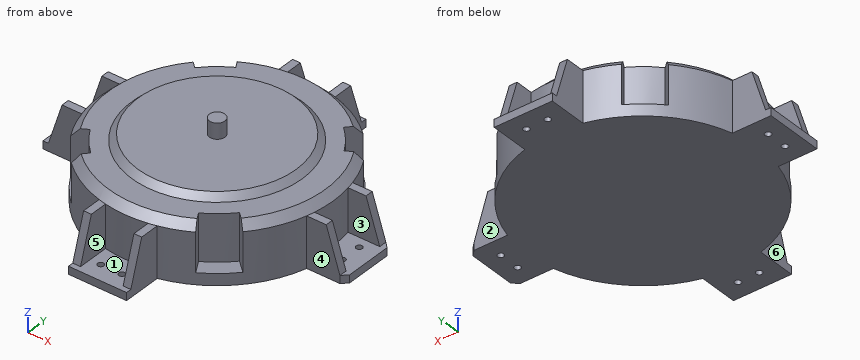
from build123d import *

# Parameters (mm, degrees)
IZIM1_R                           = 150
Y_KSEKLIK_EKSTR_ZYON1_DEPTH       = 75
PAH1_SIZE                         = 10
Y_KSEKLIK_EKSTR_ZYON2_START       = -75
Y_KSEKLIK_EKSTR_ZYON2_DEPTH       = 10
PAH2_SIZE                         = 7
Y_KSEKLIK_EKSTR_ZYON3_DEPTH       = 10
IZIM8_R                           = 4
KES_EKSTR_ZYON1_DEPTH             = 255.641782801
DAIRESEL_KAPLAMA1_COUNT           = 4
DAIRESEL_KAPLAMA1_COPY_1_DEPTH    = 10
DAIRESEL_KAPLAMA1_COPY_2_DEPTH    = 10
DAIRESEL_KAPLAMA1_COPY_3_DEPTH    = 10
DAIRESEL_KAPLAMA1_COPY_4_SKETCH_R = 4
DAIRESEL_KAPLAMA1_COPY_4_DEPTH    = 255.641782801
DAIRESEL_KAPLAMA1_COPY_5_SKETCH_R = 4
DAIRESEL_KAPLAMA1_COPY_5_DEPTH    = 255.641782801
DAIRESEL_KAPLAMA1_COPY_6_SKETCH_R = 4
DAIRESEL_KAPLAMA1_COPY_6_DEPTH    = 255.641782801
KES_EKSTR_ZYON2_START             = -60
KES_EKSTR_ZYON2_DEPTH             = 60
DAIRESEL_KAPLAMA2_COUNT           = 4
IZIM10_R                          = 110
Y_KSEKLIK_EKSTR_ZYON4_DEPTH       = 8
Y_KSEKLIK_EKSTR_ZYON4_TAPER       = 45
IZIM11_R                          = 10
Y_KSEKLIK_EKSTR_ZYON5_DEPTH       = 20


with BuildPart() as part:
    # Çizim1 → Yükseklik-Ekstrüzyon1 (new body)
    with BuildSketch(Plane.XY):
        Circle(IZIM1_R)
    extrude(amount=Y_KSEKLIK_EKSTR_ZYON1_DEPTH)

    # Pah1
    pah1_edges = [part.edges().sort_by_distance(p)[0] for p in [
        (-150, 0, 75),
    ]]
    chamfer(pah1_edges, length=PAH1_SIZE)

    # Çizim4 → Yükseklik-Ekstrüzyon2 (add)
    with BuildSketch(Plane.XY.offset(75).offset(Y_KSEKLIK_EKSTR_ZYON2_START)):
        with BuildLine():
            Line((195.236875483, -37.5), (195.236875483, 37.5))
            Line((195.236875483, 37.5), (145.236875483, 37.5))
            ThreePointArc((145.236875483, 37.5), (150, 0), (145.236875483, -37.5))
            Line((145.236875483, -37.5), (195.236875483, -37.5))
        make_face()
    y_kseklik_ekstr_zyon2 = extrude(amount=Y_KSEKLIK_EKSTR_ZYON2_DEPTH)

    # Pah2
    pah2_edges = [part.edges().sort_by_distance(p)[0] for p in [
        (195.236875483, -37.5, 5),
        (195.236875483, 37.5, 5),
    ]]
    chamfer(pah2_edges, length=PAH2_SIZE)

    # Çizim7 → Yükseklik-Ekstrüzyon3 (add)
    with BuildSketch(Plane(origin=(0, 37.5, 0), x_dir=(1, 0, 0), z_dir=(0, 1, 0))):
        Polygon((145.236875483, 0), (145.236875483, -65.015207496), (170.556875483, -65.015207496), (188.236875483, -10), (188.236875483, 0), align=None)
    y_kseklik_ekstr_zyon3 = extrude(amount=-Y_KSEKLIK_EKSTR_ZYON3_DEPTH)

    # Çizim8 → Kes-Ekstrüzyon1 (cut, through all)
    with BuildSketch(Plane.XY.offset(10)):
        with Locations((172.618437741, 13.75)):
            Circle(IZIM8_R)
    kes_ekstr_zyon1 = extrude(amount=-KES_EKSTR_ZYON1_DEPTH, mode=Mode.SUBTRACT)

    # Aynalama1: Yükseklik-Ekstrüzyon3, Kes-Ekstrüzyon1 across plane
    add(y_kseklik_ekstr_zyon3.mirror(Plane.ZX))
    add(kes_ekstr_zyon1.mirror(Plane.ZX), mode=Mode.SUBTRACT)

    # Dairesel Kaplama1: Yükseklik-Ekstrüzyon2, Yükseklik-Ekstrüzyon3, Kes-Ekstrüzyon1 ×4 about axis
    dairesel_kaplama1_axis = Axis((0, 0, 0), (0, 0, 1))
    add([y_kseklik_ekstr_zyon2.rotate(dairesel_kaplama1_axis, i * 360 / DAIRESEL_KAPLAMA1_COUNT) for i in range(1, DAIRESEL_KAPLAMA1_COUNT)])
    add([y_kseklik_ekstr_zyon3.rotate(dairesel_kaplama1_axis, i * 360 / DAIRESEL_KAPLAMA1_COUNT) for i in range(1, DAIRESEL_KAPLAMA1_COUNT)])
    add([kes_ekstr_zyon1.rotate(dairesel_kaplama1_axis, i * 360 / DAIRESEL_KAPLAMA1_COUNT) for i in range(1, DAIRESEL_KAPLAMA1_COUNT)], mode=Mode.SUBTRACT)

    # Dairesel Kaplama1 copy 1 sketch → Dairesel Kaplama1 copy 1 (add)
    with BuildSketch(Plane.YZ.offset(37.5)):
        Polygon((145.236875483, 0), (145.236875483, 65.015207496), (170.556875483, 65.015207496), (188.236875483, 10), (188.236875483, 0), align=None)
    extrude(amount=-DAIRESEL_KAPLAMA1_COPY_1_DEPTH)

    # Dairesel Kaplama1 copy 2 sketch → Dairesel Kaplama1 copy 2 (add)
    with BuildSketch(Plane(origin=(0, 37.5, 0), x_dir=(-1, 0, 0), z_dir=(0, 1, 0))):
        Polygon((145.236875483, 0), (145.236875483, 65.015207496), (170.556875483, 65.015207496), (188.236875483, 10), (188.236875483, 0), align=None)
    extrude(amount=-DAIRESEL_KAPLAMA1_COPY_2_DEPTH)

    # Dairesel Kaplama1 copy 3 sketch → Dairesel Kaplama1 copy 3 (add)
    with BuildSketch(Plane(origin=(-37.5, 0, 0), x_dir=(0, -1, 0), z_dir=(-1, 0, 0))):
        Polygon((145.236875483, 0), (145.236875483, 65.015207496), (170.556875483, 65.015207496), (188.236875483, 10), (188.236875483, 0), align=None)
    extrude(amount=-DAIRESEL_KAPLAMA1_COPY_3_DEPTH)

    # Dairesel Kaplama1 copy 4 sketch → Dairesel Kaplama1 copy 4 (cut, through all)
    with BuildSketch(Plane(origin=(0, 0, 10), x_dir=(0, 1, 0), z_dir=(0, 0, 1))):
        with Locations((172.618437741, -13.75)):
            Circle(DAIRESEL_KAPLAMA1_COPY_4_SKETCH_R)
    extrude(amount=-DAIRESEL_KAPLAMA1_COPY_4_DEPTH, mode=Mode.SUBTRACT)

    # Dairesel Kaplama1 copy 5 sketch → Dairesel Kaplama1 copy 5 (cut, through all)
    with BuildSketch(Plane(origin=(0, 0, 10), x_dir=(-1, 0, 0), z_dir=(0, 0, 1))):
        with Locations((172.618437741, -13.75)):
            Circle(DAIRESEL_KAPLAMA1_COPY_5_SKETCH_R)
    extrude(amount=-DAIRESEL_KAPLAMA1_COPY_5_DEPTH, mode=Mode.SUBTRACT)

    # Dairesel Kaplama1 copy 6 sketch → Dairesel Kaplama1 copy 6 (cut, through all)
    with BuildSketch(Plane(origin=(0, 0, 10), x_dir=(0, -1, 0), z_dir=(0, 0, 1))):
        with Locations((172.618437741, -13.75)):
            Circle(DAIRESEL_KAPLAMA1_COPY_6_SKETCH_R)
    extrude(amount=-DAIRESEL_KAPLAMA1_COPY_6_DEPTH, mode=Mode.SUBTRACT)

    # Çizim9 → Kes-Ekstrüzyon2 (cut)
    with BuildSketch(Plane.XY.offset(75).offset(KES_EKSTR_ZYON2_START)):
        with BuildLine():
            Line((-112.583302492, -65), (-129.903810568, -75))
            ThreePointArc((-129.903810568, -75), (-116.277268219, -94.760734988), (-99.673152863, -112.094882124))
            Line((-99.673152863, -112.094882124), (-86.383399148, -97.148897841))
            ThreePointArc((-86.383399148, -97.148897841), (-100.773632456, -82.125970323), (-112.583302492, -65))
        make_face()
    kes_ekstr_zyon2 = extrude(amount=KES_EKSTR_ZYON2_DEPTH, mode=Mode.SUBTRACT)

    # Dairesel Kaplama2: Kes-Ekstrüzyon2 ×4 about axis
    dairesel_kaplama2_axis = Axis((0, 0, 75), (0, 0, 1))
    for i in range(1, DAIRESEL_KAPLAMA2_COUNT):
        add(kes_ekstr_zyon2.rotate(dairesel_kaplama2_axis, i * 360 / DAIRESEL_KAPLAMA2_COUNT), mode=Mode.SUBTRACT)

    # Çizim10 → Yükseklik-Ekstrüzyon4 (add)
    with BuildSketch(Plane.XY.offset(75)):
        Circle(IZIM10_R)
    extrude(amount=Y_KSEKLIK_EKSTR_ZYON4_DEPTH, taper=Y_KSEKLIK_EKSTR_ZYON4_TAPER)

    # Çizim11 → Yükseklik-Ekstrüzyon5 (add)
    with BuildSketch(Plane.XY.offset(83)):
        Circle(IZIM11_R)
    extrude(amount=Y_KSEKLIK_EKSTR_ZYON5_DEPTH)


solid = part.part
Verification items for the finished model (mm, model axes). Face numbers are marked on the shaded views. A direction names the side the tool comes from. Round coordinates to 2 decimals unless told otherwise and drop trailing zeros. Loops run counter-clockwise (first coordinate to the right, second up) from the corner with the lowest first, then second, coordinate; pieces in that order, holes last. Notation, with made-up numbers: (38, 16) - (66, 16) arc R19 ccw to (66, 30) - close; hole circle Ø3 at (-28.75, -10). An arc over 180 degrees is marked (long way). Write item = value, one per line.
Q1. Sectioned sample at A-A on y = 0. Record the boundary of the cut face in (x, z), plus the area to 3 significant figures.
Here are the results:
outline = (-195.24, 0) - (195.24, 0) - (195.24, 10) - (150, 10) - (150, 65) - (140, 75) - (110, 75) - (102, 83) - (10, 83) - (10, 103) - (-10, 103) - (-10, 83) - (-102, 83) - (-110, 75) - (-140, 75) - (-150, 65) - (-150, 10) - (-195.24, 10) - close
area = 25,400 mm^2
Q2. Material ranges on L1, parallel to Y at x = 13.75, z = 3.5; L2, parallel to X at y = 166, z = 26.5; L3, parallel to Z at x = 91, y = -104.5, recorded low to high.
Here are the results:
L1 = -195.24 to -176.62, -168.62 to 168.62, 176.62 to 195.24
L2 = -37.5 to -27.5, 27.5 to 37.5
L3 = 0 to 15
Q3. Tool access check on the marked faces 1, 2 and 3. Record the directions out of +Z, -Z, +X, -X, +Y, -Y that give a thin tool (end or side, any length) a straight path to the whole face; none if there is none.
Here are the results:
face_1 = +Z, -Y
face_2 = +Z, -Z, +X, +Y
face_3 = +Z, +X
Q4. Depth check by flat-ended pin: pin 1 (20.5 mm diameter, centred on y = -158, z = 40.5, fed in from +X); pin 2 (10 mm diameter, centred on x = 34.5, y = 83.5, fed in from +Z); pin 3 (10 mm diameter, centred on y = 68, z = 38.5, fed in from +X); pin 4 (7 mm diameter, centred on x = 172.62, y = -13.75, fed in from -Z). Enter the tip coordinate at first touch or a pass-through.
Here are the results:
pin_1 = 37.5
pin_2 = 83
pin_3 = 136.13
pin_4 = through
Q5. Mould release check, pull along X, two halves, no side actions. Record for the marked faces 4, 5 and 6: +X half, -X half, draft (parallel to the pull), parting line (faces both ways), or undercut.
Here are the results:
face_4 = draft
face_5 = undercut
face_6 = -X half
